Here's how the part is built. I have some questions about the finished solid (model axes, mm). A direction names the side the tool comes from. Round coordinates to 2 decimals unless told otherwise and drop trailing zeros. Order: outer loops, then holes, each group sorted by start corner. A loop starts at its lowest first (then second) coordinate and runs counter-clockwise, first axis right, second up. Notation, with made-up numbers: (-5, -38.75) - (7, -38.75) arc R14 cw to (7, -31.75) - close; hole circle Ø10 at (60, 89). An arc over 180 degrees is marked (long way). Answer as a JSON object with one key per item and string values.
```python
from build123d import *

# Parameters (mm, degrees)
F0_W     = 127
F0_H     = 38.1
F1_DEPTH = 25.4
F2_W     = 115.9340298213
F2_H     = 38.1
F3_DEPTH = 25.4
F4_W     = 127
F4_H     = 68.654977391
F5_DEPTH = 25.4
F7_DEPTH = 25.4
F8_SIZE  = 5.08


# Not quite as in the source:
# - the program builds the solid bodies; features that only make, move or delete a surface that nothing else refers to are left out


with BuildPart() as f1:
    # F0 (on Top) → F1 (new body)
    with BuildSketch(Plane.XY):
        with Locations((3.9197548818, 19.05)):
            Rectangle(F0_W, F0_H)
    extrude(amount=F1_DEPTH)

    # F2 (on face) → F3 (join)
    with BuildSketch(Plane.XY.offset(25.4)):
        with Locations((9.4527399712, 19.05)):
            Rectangle(F2_W, F2_H)
    extrude(amount=F3_DEPTH)

    # F4 (on Top) → F5 (join)
    with BuildSketch(Plane.XY):
        with Locations((3.9833925518, -34.3274886955)):
            Rectangle(F4_W, F4_H)
    extrude(amount=F5_DEPTH)

    # F6 (on Top) → F7 (join)
    with BuildSketch(Plane.XY):
        Polygon((115.0657710181, -189.4061209801), (166.3690629853, 93.5014354232), (-104.2877137661, -3.5223886371), align=None)
    extrude(amount=F7_DEPTH)

    # F8
    f8_edges = [f1.edges().sort_by_distance(p)[0] for p in [
        (140.717417, -47.952343, 25.4),
        (43.819127, -129.030549, 25.4),
        (-43.472062, -68.654977, 25.4),
        (-59.516607, -55.058567, 25.4),
        (-81.902161, -22.492273, 25.4),
        (9.45274, 0, 50.8),
        (-23.879261, 38.1, 0),
        (9.45274, 38.1, 50.8),
        (67.419755, 19.05, 50.8),
        (67.419755, 0, 38.1),
        (67.419755, 19.05, 25.4),
        (67.419755, 38.1, 38.1),
        (39.620739, 38.1, 25.4),
        (9.45274, 0, 25.4),
    ]]
    chamfer(f8_edges, length=F8_SIZE)


solid = f1.part
```
1. For faces 1 (the face through (6, 0, 38)), 2 (the face through (67.42, 19, 38)), 3 (the face through (-13, 38.1, 25)), 4 (the face through (-59.517, -55, 10)), which set-ups out of +Z, -Z, +X, -X, +Y, -Y let a thin tool reach every point of the face, with its end or its side?
Responses:
{"face 1": "+Z, +X, -X, -Y", "face 2": "+Z, +X, +Y, -Y", "face 3": "+Z, -X, +Y", "face 4": "+Z, -Z, -X, -Y"}
2. Imagine slicing it at B-B (z = 11.5). List the corners of the cut face in (x, y) for me.
Responses:
{"outline": "(-104.29, -3.52) - (-59.52, -41.46) - (-59.52, -68.65) - (-27.43, -68.65) - (115.07, -189.41) - (166.37, 93.5) - (11.82, 38.1) - (-59.58, 38.1) - (-59.58, 12.5) - close"}
3. Imagine slicing it at C-C (y = -120). List the corners of the cut face in (x, z) for me.
Responses:
{"outline": "(33.16, 0) - (127.65, 0) - (127.65, 20.32) - (122.49, 25.4) - (41.02, 25.4) - (33.16, 20.32) - close"}
4. If I drill on L1, parallel to Y at x = 57, z = 32.5; L2, parallel to Y at x = -48.5, z = 7.5; L3, parallel to Z at x = 119, y = 3.5, over which ranges is the centre line in solid material (lowest first)? Write a range as [from, to].
Responses:
{"L1": "[0, 38.1]", "L2": "[-68.65, 38.1]", "L3": "[0, 25.4]"}
5. Imagine slicing it at A-A (x = -31.5). List the corners of the cut face in (y, z) for me.
Responses:
{"outline": "(-68.65, 0) - (33.02, 0) - (38.1, 5.08) - (38.1, 45.72) - (33.02, 50.8) - (5.08, 50.8) - (0, 45.72) - (0, 30.48) - (-5.08, 25.4) - (-63.57, 25.4) - (-68.65, 20.32) - close"}
6. Imagine slicing it at D-D (z = 37). List the corners of the cut face in (x, y) for me.
Responses:
{"outline": "(-48.51, 0) - (62.34, 0) - (67.42, 5.08) - (67.42, 33.02) - (62.34, 38.1) - (-48.51, 38.1) - close"}
7. For P1, Ø8, axis at x = 35.5, y = -1, coming from the +Z side; P2, Ø1.5, axis at y = 12.5, z = 41, coming from the -X side; P3, Ø10, axis at y = -19, z = 17, coming from the -X side, each with a flat end and sliding along its axis, tell me the tip position at first contact or that it passes through.
Responses:
{"P1": "z = 48.72", "P2": "x = -48.51", "P3": "x = -91.92"}
